Source: CAD feature listing. Evaluate the final solid. Frame: model axes, mm. Round coordinates to 2 decimals unless told otherwise and drop trailing zeros. Loops run counter-clockwise (first coordinate to the right, second up) from the corner with the lowest first, then second, coordinate; pieces in that order, holes last. Notation, with made-up numbers: (39, -28) -> (52, -28) arc R19 cw to (52, -1) -> close; hole circle Ø5 at (8, -17.75). An arc over 180 degrees is marked (long way). Return JSON: item names as keys, results as strings. Group by question number.
```python
from build123d import *

# Parameters (mm, degrees)
SKETCH1_R           = 7.5
SKETCH1_R_2         = 4
BOSS_EXTRUDE1_DEPTH = 24
SKETCH2_R           = 0.5


with BuildPart() as part:
    # Sketch1 → Boss-Extrude1 (new body)
    with BuildSketch(Plane(origin=(0, 0, 0), x_dir=(1, 0, 0), z_dir=(0, 1, 0))):
        Circle(SKETCH1_R)
        Circle(SKETCH1_R_2, mode=Mode.SUBTRACT)
    extrude(amount=BOSS_EXTRUDE1_DEPTH)

    # Sketch2 → Cut-Revolve1 (revolve, cut)
    with BuildSketch(Plane.XY):
        with Locations((7.5, 4)):
            Circle(SKETCH2_R)
        with Locations((7.5, 20)):
            Circle(SKETCH2_R)
    revolve(axis=Axis((0, 20.782039023, 0), (0, -1, 0)), mode=Mode.SUBTRACT)


solid = part.part
```
(1) Cut plane A-A (z = 0). Return loops of the section in (x, y).
(2) Ray query, line 1 (X direction, y = 9.5, z = 0); line 2 (X direction, y = 12.75, z = -1.75). Return the intervals inside material, ascending.
(3) Cut plane B-B (x = 0). Return loops of the section in (y, z), and give its area (3 significant figures).
(4) Pin query (flat end, axial travel): pin 1 (1 mm diameter, centred on y = 15.5, z = 1, fed in from +X); pin 2 (1 mm diameter, centred on y = 19.5, z = -2.5, fed in from -X); pin 3 (4 mm diameter, centred on y = 11, z = -3, fed in from +X). Return the tip coordinate at first contact, or that it passes through.
(5) Cut plane C-C (y = 14.75). Return loops of the section in (x, z), and give its area (3 significant figures).
Answers follow:
{
 "1": {"outline": "(-7.5, 0) -> (-4, 0) -> (-4, 24) -> (-7.5, 24) -> (-7.5, 20.5) arc R0.5 cw to (-7.5, 19.5) -> (-7.5, 4.5) arc R0.5 cw to (-7.5, 3.5) -> close; (4, 0) -> (7.5, 0) -> (7.5, 3.5) arc R0.5 cw to (7.5, 4.5) -> (7.5, 19.5) arc R0.5 cw to (7.5, 20.5) -> (7.5, 24) -> (4, 24) -> close"},
 "2": {"line 1": "-7.5 to -4, 4 to 7.5", "line 2": "-7.29 to -3.6, 3.6 to 7.29"},
 "3": {"outline": "(0, -7.5) -> (3.5, -7.5) arc R0.5 cw to (4.5, -7.5) -> (19.5, -7.5) arc R0.5 cw to (20.5, -7.5) -> (24, -7.5) -> (24, -4) -> (0, -4) -> close; (0, 4) -> (24, 4) -> (24, 7.5) -> (20.5, 7.5) arc R0.5 cw to (19.5, 7.5) -> (4.5, 7.5) arc R0.5 cw to (3.5, 7.5) -> (0, 7.5) -> close", "area": "166 mm^2"},
 "4": {"pin 1": "x = 7.48", "pin 2": "x = -7.23", "pin 3": "x = 7.43"},
 "5": {"outline": "circle Ø15 at (0, 0); hole circle Ø8 at (0, 0)", "area": "126 mm^2"}
}
